from build123d import *

# Parameters (mm, degrees)
F1_DEPTH = 25.4
F2_DEPTH = 12.7
F0_W     = 50.8
F0_H     = 12.7
F3_DEPTH = 38.1
F4_R     = 6.35
F5_DEPTH = 12.701
F6_R     = 5.08


with BuildPart() as f1:
    # F0 (on Front) → F1 (new body)
    with BuildSketch(Plane.XZ):
        with BuildLine():
            ThreePointArc((0, 57.254138), (-12.7, 69.954138), (-25.4, 57.254138))
            Line((-25.4, 57.254138), (-19.05, 57.254138))
            ThreePointArc((-19.05, 57.254138), (-12.7, 63.604138), (-6.35, 57.254138))
            Line((-6.35, 57.254138), (0, 57.254138))
        make_face()
        with BuildLine():
            Line((-19.05, 57.254138), (-25.4, 57.254138))
            ThreePointArc((-25.4, 57.254138), (-12.7, 44.554138), (0, 57.254138))
            Line((0, 57.254138), (-6.35, 57.254138))
            ThreePointArc((-6.35, 57.254138), (-12.7, 50.904138), (-19.05, 57.254138))
        make_face()
    extrude(amount=F1_DEPTH)

    # F0 (on Front) → F2 (join)
    with BuildSketch(Plane.XZ):
        with BuildLine():
            ThreePointArc((-25.4, 25.504138), (-29.082574, 16.456638), (-38.099573, 12.7))
            Line((-38.099573, 12.7), (12.700427, 12.7))
            ThreePointArc((12.700427, 12.7), (3.682874, 16.456335), (0, 25.504138))
            Line((0, 25.504138), (0, 57.254138))
            ThreePointArc((0, 57.254138), (-12.7, 44.554138), (-25.4, 57.254138))
            Line((-25.4, 57.254138), (-25.4, 25.504138))
        make_face()
    extrude(amount=F2_DEPTH)

    # F0 (on Front) → F3 (join)
    with BuildSketch(Plane.XZ):
        with Locations((-12.699573, 6.35)):
            Rectangle(F0_W, F0_H)
    extrude(amount=F3_DEPTH)

    # F4 (on face) → F5 (cut, through all)
    with BuildSketch(Plane.XY.offset(12.7)):
        with Locations((-12.7, -25.4)):
            Circle(F4_R)
    extrude(amount=-F5_DEPTH, mode=Mode.SUBTRACT)

    # F6
    f6_edges = [f1.edges().sort_by_distance(p)[0] for p in [
        (12.700427, -38.1, 6.35),
        (-38.099573, -38.1, 6.35),
    ]]
    fillet(f6_edges, radius=F6_R)


solid = f1.part
Geometry: final body of the model. Coordinates: model frame, mm. A direction names the side the tool comes from. Give positions to 0.01 mm unless a question says otherwise; leave off trailing zeros. Loops run counter-clockwise (first coordinate to the right, second up) from the corner with the lowest first, then second, coordinate; pieces in that order, holes last. Notation, with made-up numbers: (4, -38.5) - (15, -38.5) arc R21 cw to (15, -8.5) - close; hole circle Ø6 at (-7.5, 50). An arc over 180 degrees is marked (long way). One line per question, with ' | ' between items. Start each with the question number.
(1) Pull-direction query (Z, two-part tool) for faces 1 (the flat face through (-19, -28, 12.7)), 2 (the flat face through (-13.1, -18.8, 0)), 3 (the flat face through (-13, 0, 28)); classes: released by +Z, released by -Z, zero draft, split by the parting line, or undercut.
(2) Section query D-D on x = -22. Return loops of the section in (y, z), then the cut area to 3 significant figures.
(3) Section query A-A on y = -18. Return loops of the section in (x, z).
(4) Section query B-B on x = -12.7. Return loops of the section in (y, z).
(5) Contact query for flat-ended pins moving along their axis: pin 1 (6.5 mm diameter, centred on y = -5.5, z = 48, fed in from +X); pin 2 (14 mm diameter, centred on y = -7, z = 42, fed in from -X); pin 3 (6 mm diameter, centred on x = -4, z = 47, fed in from -Y). Output: stop coordinate, or through.
(6) Reachability of faces 4 (the flat face through (-19, -25.4, 55)), 5 (the cylindrical face through (-9.77, -31.034, 6.439)), 6 (the flat face through (-25.4, -6, 42)), 7 (the cylindrical face through (-18.6, -15.3, 68.5)), 8 (the flat face through (0, -6, 41)) from +Z, -Z, +X, -X, +Y, -Y: full face, straight path, thin tool, end or side. Return the list, or none.
(7) Ray query, line 1 (Z direction, x = -12.7, y = -16.25); line 2 (Y direction, x = -12.7, z = 8.25); line 3 (Z direction, x = -12.7, y = -12). Return the intervals inside material, ascending. Write a range as from..to.
(8) Section query C-C on z = 4. Return loops of the section in (x, y), then the cut area to 3 significant figures.
The answers:
1) face 1: undercut | face 2: released by -Z | face 3: zero draft
2) outline: (-38.1, 0) - (0, 0) - (0, 65.9) - (-25.4, 65.9) - (-25.4, 48.61) - (-12.7, 48.61) - (-12.7, 12.7) - (-38.1, 12.7) - close | area: 1,380 mm2
3) outline: (-38.1, 0) - (12.7, 0) - (12.7, 12.7) - (-38.1, 12.7) - close; circle Ø25.4 at (-12.7, 57.25); hole circle Ø12.7 at (-12.7, 57.25)
4) outline: (-38.1, 0) - (-31.75, 0) - (-31.75, 12.7) - (-38.1, 12.7) - close; (-25.4, 44.55) - (-12.7, 44.55) - (-12.7, 12.7) - (-19.05, 12.7) - (-19.05, 0) - (0, 0) - (0, 50.9) - (-25.4, 50.9) - close; (-25.4, 63.6) - (0, 63.6) - (0, 69.95) - (-25.4, 69.95) - close
5) pin 1: x = 0 | pin 2: x = -25.4 | pin 3: y = -25.4
6) face 4: +Z, +X, -X, -Y | face 5: -Z | face 6: +Z, -X, +Y, -Y | face 7: -Y | face 8: +Z, +X, +Y, -Y
7) line 1: 0..12.7, 44.55..50.9, 63.6..69.95 | line 2: -38.1..-31.75, -19.05..0 | line 3: 0..50.9, 63.6..69.95
8) outline: (-38.1, -33.02) arc R5.08 ccw to (-33.02, -38.1) - (7.62, -38.1) arc R5.08 ccw to (12.7, -33.02) - (12.7, 0) - (-38.1, 0) - close; hole circle Ø12.7 at (-12.7, -25.4) | area: 1,800 mm2
